from build123d import *

# Parameters (mm, degrees)
SCHIZZO1_W                   = 9
SCHIZZO1_H                   = 4
ESTRUSIONE_ESTRUSIONE1_DEPTH = 4
SCHIZZO2_W                   = 4
SCHIZZO2_H                   = 6.25
ESTRUSIONE_ESTRUSIONE2_DEPTH = 4
RIPETIZIONE_A_L1_COUNT       = 4
RIPETIZIONE_A_L1_PITCH       = 12.5


with BuildPart() as part:
    # Schizzo1 → Estrusione-Estrusione1 (new body)
    with BuildSketch(Plane.XY):
        Polygon((0, 50), (-23.8, 20.3), (-23.8, 0.3), (0, -2), align=None)
        with Locations((-12.3, 5.67)):
            Rectangle(SCHIZZO1_W, SCHIZZO1_H, mode=Mode.SUBTRACT)
        with Locations((-12.3, 14.93)):
            Rectangle(SCHIZZO1_W, SCHIZZO1_H, mode=Mode.SUBTRACT)
    extrude(amount=ESTRUSIONE_ESTRUSIONE1_DEPTH)

    # Schizzo2 → Estrusione-Estrusione2 (add)
    with BuildSketch(Plane.XY.offset(4)):
        with Locations((2, 43.75)):
            Rectangle(SCHIZZO2_W, SCHIZZO2_H)
    estrusione_estrusione2 = extrude(amount=-ESTRUSIONE_ESTRUSIONE2_DEPTH)

    # Ripetizione a L1: Estrusione-Estrusione2 ×4
    with Locations(*[(0, -i * RIPETIZIONE_A_L1_PITCH, 0) for i in range(1, RIPETIZIONE_A_L1_COUNT)]):
        add(estrusione_estrusione2)


solid = part.part
Build history of the part. All positions in model axes, mm. A direction names the side the tool comes from. Coordinates: 2 decimals unless noted, no trailing zeros. Write each loop counter-clockwise with the first axis right and the second up, starting at its lowest first coordinate (ties: lowest second). Pieces come first, ordered by that corner, then holes. Notation, with made-up numbers: (-4, -25) -> (16, -25) arc R11 ccw to (16, -21) -> close; hole circle Ø2 at (-34, 17). An arc over 180 degrees is marked (long way). Use CSV: the item, a comma, the result in double quotes. Start each with the question number.
Q1. Cut at C-C, the plane z = 3.4. List the corners of the cut face in (x, y) (3 decimals), then the cut area to 3 significant figures.
Q2. Drill centre lines: probe 1 along Y at (x, z) = (-13, 3.35); probe 2 along Y at (x, z) = (-8, 1.6); probe 3 along X at (y, z) = (9.5, 0.75). Where is each one in solid material? Low to high.
Q3. Cut at D-D, the plane x = -8.5. List the corners of the cut face in (y, z), then the cut area to 3 significant figures.
Q4. Cut at A-A, the plane x = 0.5. List the corners of the cut face in (y, z) (3 decimals), then the cut area to 3 significant figures.
Q5. Flat gauge pins, fed straight in: pin 1 Ø10 at (x, y) = (-3.5, 34.5) entering from -Z; pin 2 Ø1.5 at (y, z) = (25.5, 3.5) entering from +X; pin 3 Ø1.2 at (x, z) = (2, 2) entering from +Y (3 decimals); pin 4 Ø2 at (x, z) = (-13.5, 3) entering from +Y. Where does each tip first touch, or does it go through?
Q6. 3-axis set-ups, long thin cutter, end or side, ignore diameter. For faces 1 (the flat face through (-12, 7.67, 2)), 2 (the flat face through (2, 9.375, 2)), 3 (the flat face through (2, 46.875, 2)): which of +Z, -Z, +X, -X, +Y, -Y reach the whole face in a straight line?
Q7. Pull direction Y, two halves, no side cores. Call faces 4 (the flat face through (-12.067, -0.834, 1.972)), 5 (the flat face through (-10, 19, 4)), 6 (the flat face through (0, 37, 2)): released by +Y, released by -Y, zero draft, split by the parting line, or undercut.
Q8. Cut at B-B, the plane x = -12.25. List the corners of the cut face in (y, z).
Checked values:
1,outline,"(-23.8, 0.3) -> (0, -2) -> (0, 3.125) -> (4, 3.125) -> (4, 9.375) -> (0, 9.375) -> (0, 15.625) -> (4, 15.625) -> (4, 21.875) -> (0, 21.875) -> (0, 28.125) -> (4, 28.125) -> (4, 34.375) -> (0, 34.375) -> (0, 40.625) -> (4, 40.625) -> (4, 46.875) -> (0, 46.875) -> (0, 50) -> (-23.8, 20.3) -> close; hole (-16.8, 3.67) -> (-7.8, 3.67) -> (-7.8, 7.67) -> (-16.8, 7.67) -> close; hole (-16.8, 12.93) -> (-7.8, 12.93) -> (-7.8, 16.93) -> (-16.8, 16.93) -> close"
1,area,"885 mm²"
2,probe 1,"y = -0.74 to 3.67, 7.67 to 12.93, 16.93 to 33.78"
2,probe 2,"y = -1.23 to 3.67, 7.67 to 12.93, 16.93 to 40.02"
2,probe 3,"x = -23.8 to 0"
3,outline,"(-1.18, 0) -> (3.67, 0) -> (3.67, 4) -> (-1.18, 4) -> close; (7.67, 0) -> (12.93, 0) -> (12.93, 4) -> (7.67, 4) -> close; (16.93, 0) -> (39.39, 0) -> (39.39, 4) -> (16.93, 4) -> close"
3,area,"130 mm²"
4,outline,"(3.125, 0) -> (9.375, 0) -> (9.375, 4) -> (3.125, 4) -> close; (15.625, 0) -> (21.875, 0) -> (21.875, 4) -> (15.625, 4) -> close; (28.125, 0) -> (34.375, 0) -> (34.375, 4) -> (28.125, 4) -> close; (40.625, 0) -> (46.875, 0) -> (46.875, 4) -> (40.625, 4) -> close"
4,area,"100 mm²"
5,pin 1,"stops at z = 0"
5,pin 2,"stops at x = 0"
5,pin 3,"stops at y = 46.875"
5,pin 4,"stops at y = 34.4"
6,face 1,"+Z, -Z"
6,face 2,"+Z, -Z, +X"
6,face 3,"+Z, -Z, +X, +Y"
7,face 4,"released by -Y"
7,face 5,"zero draft"
7,face 6,"undercut"
8,outline,"(-0.82, 0) -> (3.67, 0) -> (3.67, 4) -> (-0.82, 4) -> close; (7.67, 0) -> (12.93, 0) -> (12.93, 4) -> (7.67, 4) -> close; (16.93, 0) -> (34.71, 0) -> (34.71, 4) -> (16.93, 4) -> close"
